Model file for the job. Use its own axes, mm. Face numbers are marked on the shaded views. A direction names the side the tool comes from. Give positions to 0.01 mm unless a question says otherwise; leave off trailing zeros. Write each loop counter-clockwise with the first axis right and the second up, starting at its lowest first coordinate (ties: lowest second). Pieces come first, ordered by that corner, then holes. Notation, with made-up numbers: (76, 39.25) - (106, 39.25) arc R30 cw to (106, 72.25) - close; hole circle Ø1 at (17.25, 8.5). An arc over 180 degrees is marked (long way). One line per item, written item: value. Start each with the question number.
(1) Cut at D-D, the plane x = -37.5. List the corners of the cut face in (y, z), and give its area (3 significant figures).
(2) Probe L1, parallel to Y at x = -10, z = 31.5. List the from-to ranges inside material, lowest first.
(3) 3-axis set-ups, long thin cutter, end or side, ignore diameter. For the marked faces 1, 2 and 3: which of +Z, -Z, +X, -X, +Y, -Y reach the whole face in a straight line?
(4) Cut at C-C, the plane y = -63.5. List the corners of the cut face in (x, z), and give its area (3 significant figures).
(5) Drop flat-ended pins along their axis: P1, Ø6.5, axis at x = -55.5, y = -66, coming from the -Z side; P2, Ø10, axis at y = -69, z = 47, coming from the +X side; P3, Ø2, axis at x = -20, z = 69.5, coming from the -Y side. Give the stop position or say it passes through.
(6) Cut at B-B, the plane z = 45.5. List the corners of the cut face in (x, y).
(7) Cut at A-A, the plane x = -61. List the corners of the cut face in (y, z).
from build123d import *

# Parameters (mm, degrees)
F0_W      = 76.2
F0_H      = 76.2
F1_DEPTH  = 25.4
F1_FACE_W = 76.2
F1_FACE_H = 76.2
F2_DEPTH  = 35.306
F4_DEPTH  = 12.7


with BuildPart() as f1:
    # F0 (on Front) → F1 (new body)
    with BuildSketch(Plane.XZ):
        with Locations((-38.1, 41.869526)):
            Rectangle(F0_W, F0_H)
    extrude(amount=F1_DEPTH)

    # F0 (on Front) + F1_face (on face) → F2 (join)
    with BuildSketch(Plane.XZ):
        with Locations((-38.1, 41.869526)):
            Rectangle(F0_W, F0_H)
    with BuildSketch(Plane(origin=(-38.1, -25.4, 41.869526), x_dir=(1, 0, 0), z_dir=(0, -1, 0))):
        Rectangle(F1_FACE_W, F1_FACE_H)
    extrude(amount=F2_DEPTH)

    # F3 (on face) → F4 (join)
    with BuildSketch(Plane.XZ.offset(60.706)):
        Polygon((-44.259132, 29.169526), (-44.259132, 54.569526), (-56.959132, 54.569526), (-60.402479, 54.569526), (-69.659132, 54.569526), (-69.659132, 29.169526), align=None)
    extrude(amount=F4_DEPTH)


solid = f1.part
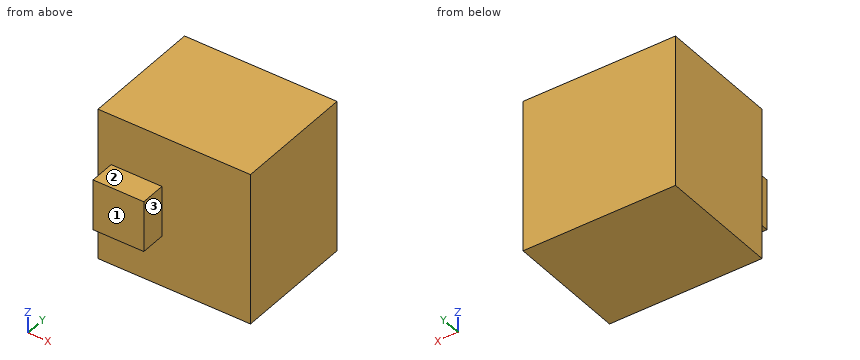
Answers follow:
1. outline: (-60.71, 3.77) - (0, 3.77) - (0, 79.97) - (-60.71, 79.97) - close
1. area: 4,630 mm²
2. L1: y = -60.71 to 0
3. face 1: +Z, -Z, +X, -X, -Y
3. face 2: +Z, +X, -X, -Y
3. face 3: +Z, -Z, +X, -Y
4. outline: (-69.66, 29.17) - (-44.26, 29.17) - (-44.26, 54.57) - (-69.66, 54.57) - close
4. area: 645 mm²
5. P1: stops at z = 29.17
5. P2: stops at x = -44.26
5. P3: stops at y = -60.71
6. outline: (-76.2, -60.71) - (-69.66, -60.71) - (-69.66, -73.41) - (-44.26, -73.41) - (-44.26, -60.71) - (0, -60.71) - (0, 0) - (-76.2, 0) - close
7. outline: (-73.41, 29.17) - (-60.71, 29.17) - (-60.71, 3.77) - (0, 3.77) - (0, 79.97) - (-60.71, 79.97) - (-60.71, 54.57) - (-73.41, 54.57) - close
